The model under review builds one solid part; all positions refer to its coordinate system, in mm. A direction names the side the tool comes from. Give positions to 0.01 mm unless a question says otherwise; leave off trailing zeros. Write each loop counter-clockwise with the first axis right and the second up, starting at its lowest first coordinate (ties: lowest second). Pieces come first, ordered by that corner, then holes. Notation, with made-up numbers: (-39, 21.5) -> (-31, 21.5) arc R14 cw to (-31, 43.5) -> close; hole circle Ø2 at (29.5, 19.25). An arc over 180 degrees is marked (long way). Use CSV: the item, a comma, the result in double quotes.
```python
from build123d import *

# Parameters (mm, degrees)
SKETCH1_R           = 2.25
SKETCH1_W           = 6.5
SKETCH1_H           = 10.7
BOSS_EXTRUDE1_DEPTH = 2
SKETCH3_W           = 4
SKETCH3_H           = 15
BOSS_EXTRUDE2_DEPTH = 16
FILLET1_R           = 10
FILLET2_R           = 4
CHAMFER1_SIZE       = 3
CHAMFER1_SIZE2      = 5.196152423
CUT_EXTRUDE2_DEPTH  = 16
SKETCH10_R          = 2.468429883
SKETCH10_R_2        = 1.75
SKETCH10_W          = 3.2
SKETCH10_H          = 15
CUT_EXTRUDE3_DEPTH  = 4
SKETCH12_W          = 53.277727804
SKETCH12_H          = 68.29561081
CUT_EXTRUDE4_DEPTH  = 23


with BuildPart() as part:
    # Sketch1 → Boss-Extrude1 (new body, symmetric)
    with BuildSketch(Plane(origin=(0, -35, 0), x_dir=(1, 0, 0), z_dir=(0, 1, 0))):
        with BuildLine():
            Line((-50, 76.225749335), (50, 76.225749335))
            ThreePointArc((50, 76.225749335), (53.535533906, 74.761283241), (55, 71.225749335))
            Line((55, 71.225749335), (55, -3.774250665))
            Line((55, -3.774250665), (20.347942177, -78.774250665))
            Line((20.347942177, -78.774250665), (20.347942177, -82.95646352))
            ThreePointArc((20.347942177, -82.95646352), (21.812408271, -86.491997426), (25.347942177, -87.95646352))
            Line((25.347942177, -87.95646352), (63.43950887, -87.95646352))
            ThreePointArc((63.43950887, -87.95646352), (66.133427762, -87.168683956), (67.978460954, -85.053583921))
            Line((67.978460954, -85.053583921), (73.038309614, -74.102180936))
            Line((73.038309614, -74.102180936), (80.685361178, -83.086313097))
            ThreePointArc((80.685361178, -83.086313097), (82.977793564, -88.210367772), (82.148282135, -93.762222718))
            Line((82.148282135, -93.762222718), (77.534981649, -103.747128614))
            ThreePointArc((77.534981649, -103.747128614), (75.219554646, -106.919630821), (71.860949779, -108.955741281))
            Line((71.860949779, -108.955741281), (9.40285347, -131.565833476))
            Line((9.40285347, -131.565833476), (-9.40285347, -131.565833476))
            Line((-9.40285347, -131.565833476), (-71.860949779, -108.955741281))
            ThreePointArc((-71.860949779, -108.955741281), (-75.219554646, -106.919630821), (-77.534981649, -103.747128614))
            Line((-77.534981649, -103.747128614), (-82.148282135, -93.762222718))
            ThreePointArc((-82.148282135, -93.762222718), (-82.977793564, -88.210367772), (-80.685361178, -83.086313097))
            Line((-80.685361178, -83.086313097), (-73.038309614, -74.102180936))
            Line((-73.038309614, -74.102180936), (-67.978460954, -85.053583921))
            ThreePointArc((-67.978460954, -85.053583921), (-66.133427762, -87.168683956), (-63.43950887, -87.95646352))
            Line((-63.43950887, -87.95646352), (-25.347942177, -87.95646352))
            ThreePointArc((-25.347942177, -87.95646352), (-21.812408271, -86.491997426), (-20.347942177, -82.95646352))
            Line((-20.347942177, -82.95646352), (-20.347942177, -78.774250665))
            Line((-20.347942177, -78.774250665), (-55, -3.774250665))
            Line((-55, -3.774250665), (-55, 71.225749335))
            ThreePointArc((-55, 71.225749335), (-53.535533906, 74.761283241), (-50, 76.225749335))
        make_face()
        with Locations((-37.233481524, -94.993785432)):
            Circle(SKETCH1_R, mode=Mode.SUBTRACT)
        with Locations((37.266518397, -94.993786505)):
            Circle(SKETCH1_R, mode=Mode.SUBTRACT)
        with Locations((-52.183481524, -99.643785432)):
            Rectangle(SKETCH1_W, SKETCH1_H, mode=Mode.SUBTRACT)
        with Locations((-22.183481524, -99.643785432)):
            Rectangle(SKETCH1_W, SKETCH1_H, mode=Mode.SUBTRACT)
        with Locations((22.316518476, -99.643785432)):
            Rectangle(SKETCH1_W, SKETCH1_H, mode=Mode.SUBTRACT)
        with Locations((54.016518476, -100.243785432)):
            Rectangle(SKETCH1_W, SKETCH1_H, mode=Mode.SUBTRACT)
        with Locations((0, -113.343785432)):
            Rectangle(SKETCH1_W, SKETCH1_H, mode=Mode.SUBTRACT)
    extrude(amount=BOSS_EXTRUDE1_DEPTH, both=True)

    # Sketch3 → Boss-Extrude2 (add)
    with BuildSketch(Plane.XZ.offset(37)):
        with Locations((0, 80.45646352)):
            Rectangle(SKETCH3_W, SKETCH3_H)
    extrude(amount=BOSS_EXTRUDE2_DEPTH)

    # Fillet1
    fillet1_edges = [part.edges().sort_by_distance(p)[0] for p in [
        (0, -53, 87.95646352),
    ]]
    fillet(fillet1_edges, radius=FILLET1_R)

    # Fillet2
    fillet2_edges = [part.edges().sort_by_distance(p)[0] for p in [
        (0, -53, 72.95646352),
    ]]
    fillet(fillet2_edges, radius=FILLET2_R)

    # Chamfer1
    chamfer1_edges = [part.edges().sort_by_distance(p)[0] for p in [
        (0, -37, 87.95646352),
        (-2, -37, 80.45646352),
        (0, -37, 72.95646352),
        (2, -37, 80.45646352),
    ]]
    chamfer1_side = [part.faces().sort_by_distance(p)[0] for p in [
        (-0.006927699, -37, 22.010129075),
    ]]
    chamfer(chamfer1_edges, length=CHAMFER1_SIZE, length2=CHAMFER1_SIZE2, reference=chamfer1_side[0])

    # Sketch7 → Cut-Extrude2 (cut)
    with BuildSketch(Plane.ZY.offset(2)):
        with BuildLine():
            add(Edge.make_bspline(
                [(72.95646352, -42.196152423), (75.352950237, -47.994562928), (72.95646352, -49)],
                knots=[0, 0, 0, 0.704450442, 0.704450442, 0.704450442], degree=2))
            Line((72.95646352, -42.196152423), (72.95646352, -49))
        make_face()
    extrude(amount=-CUT_EXTRUDE2_DEPTH, mode=Mode.SUBTRACT)

    # Sketch10 → Cut-Extrude3 (cut)
    with BuildSketch(Plane.XZ.offset(37)):
        with Locations((-9.838945551, -29.868495219)):
            Circle(SKETCH10_R)
        with Locations((9.838945551, -29.868495219)):
            Circle(SKETCH10_R)
        with Locations((-37.673971089, 6.665090314)):
            Circle(SKETCH10_R_2)
        with Locations((-26.592001418, -67.180357374)):
            Circle(SKETCH10_R_2)
        with Locations((37.673971089, 6.665090314)):
            Circle(SKETCH10_R_2)
        with Locations((26.592001418, -67.180357374)):
            Circle(SKETCH10_R_2)
        with Locations((-53.4, -35.847350079)):
            Rectangle(SKETCH10_W, SKETCH10_H)
        with Locations((-31.047145488, -35.847350079)):
            Rectangle(SKETCH10_W, SKETCH10_H)
        with Locations((31.047145488, -35.847350079)):
            Rectangle(SKETCH10_W, SKETCH10_H)
        with Locations((53.4, -35.847350079)):
            Rectangle(SKETCH10_W, SKETCH10_H)
    extrude(amount=-CUT_EXTRUDE3_DEPTH, mode=Mode.SUBTRACT)

    # Sketch12 → Cut-Extrude4 (cut)
    with BuildSketch(Plane(origin=(0, -37, 0), x_dir=(-1, 0, 0), z_dir=(0, -1, 0))):
        with Locations((0.715137286, -79.433896391)):
            Rectangle(SKETCH12_W, SKETCH12_H)
    extrude(amount=CUT_EXTRUDE4_DEPTH, mode=Mode.SUBTRACT)


solid = part.part
```
Q1. Insertion check: pin 1 (1.2 mm diameter, centred on y = -36, z = -64, fed in from +X); pin 2 (2 mm diameter, centred on y = -35.5, z = 101.5, fed in from -X); pin 3 (1 mm diameter, centred on x = -28, y = -35, fed in from +Z). Each pin has a flat end and moves straight along its axis. Give the tip position at first contact, or say it passes through.
Derived:
pin 1,"stops at x = 55"
pin 2,"stops at x = -79.04"
pin 3,"stops at z = 125.01"
Q2. To check wall thickness, follow probe 1 along Z at (x, y) = (1, -35); probe 2 along X at (y, z) = (-34.35, 103); probe 3 along X at (y, z) = (-36.25, 0.5). State the ranges of each line that lie inside material, in increasing order.
Derived:
probe 1,"z = -76.23 to 107.99, 118.69 to 131.57"
probe 2,"x = -77.88 to -55.43, -48.93 to -25.43, -18.93 to 19.07, 25.57 to 50.77, 57.27 to 77.88"
probe 3,"x = -55 to 55"
Q3. The part is to be moulded in two halves that separate along Z. For faces 1 (the flat face through (50.767, -35, 100)), 2 (the flat face through (0, -35, 131.566)), 3 (the cylindrical face through (-53.574, -34.972, -74.722)), say which applies: pulls with the +Z half, pulls with the -Z half, needs draft (parallel to the pull), parting line crosses it, or undercut.
Derived:
face 1,"undercut"
face 2,"pulls with the +Z half"
face 3,"pulls with the -Z half"
Q4. Machinability: for faces 4 (the cylindrical face through (21.77, -34.97, 86.45)), 5 (the cylindrical face through (-66.167, -34.972, 87.147)), 6 (the flat face through (51.8, -35, -36)), which of the approach directions +Z, -Z, +X, -X, +Y, -Y give a long, thin tool a straight path to every point of the face, cutting with its end or side? Answer none if there is none.
Derived:
face 4,"+Y, -Y"
face 5,"-Z, +Y, -Y"
face 6,"+X, +Y, -Y"
Q5. Consider section C-C (y = -35.65). State how many separate pieces and enclosed holes the cut face has, then the cut area to 3 significant figures.
Derived:
separate pieces,"1"
enclosed holes,"15"
area,"19,600 mm2"
Q6. Consider section A-A (z = -39.5). Write out the cut boundary in (x, y), then the cut area to 3 significant figures.
Derived:
outline,"(-51.8, -37) -> (-32.65, -37) -> (-32.65, -33) -> (-51.8, -33) -> close; (-29.45, -37) -> (29.45, -37) -> (29.45, -33) -> (-29.45, -33) -> close; (32.65, -37) -> (51.8, -37) -> (51.8, -33) -> (32.65, -33) -> close"
area,"389 mm2"
Q7. Consider section D-D (z = 66). Write out the cut boundary in (x, y), then the cut area to 3 significant figures.
Derived:
outline,"(-26.25, -37) -> (26.25, -37) -> (26.25, -33) -> (-26.25, -33) -> close"
area,"210 mm2"
Q8. Consider section B-B (x = -43.5). Write out the cut boundary in (y, z).
Derived:
outline,"(-37, -76.23) -> (-33, -76.23) -> (-33, 28.66) -> (-37, 28.66) -> close; (-37, 87.96) -> (-33, 87.96) -> (-33, 119.22) -> (-37, 119.22) -> close"
